```python
from build123d import *

# Parameters (mm, degrees)
F0_W        = 630
F0_H        = 480
F0_R        = 196.5
F1_DEPTH    = 22
F2_T1_DEPTH = 774.568322948
F3_SIZE     = 5


# Not quite as in the source:
# - a fillet or chamfer that OpenCascade refuses, or shapes differently, is made with other operations: its cross-section is extruded or revolved along the edge and cut away or added


with BuildPart() as f1:
    # F0 (on Front) → F1 (new body)
    with BuildSketch(Plane.XZ):
        Rectangle(F0_W, F0_H)
        with Locations((0, -15)):
            Circle(F0_R, mode=Mode.SUBTRACT)
    extrude(amount=F1_DEPTH)

    # F2: fillet of radius 30 on 1 edges, made by hand

    # F2_s2 → F2_t1 (cut)
    with BuildSketch(Plane.YZ.offset(-387.284161474)):
        with BuildLine():
            ThreePointArc((0, 240), (-15.8746727726, 229.252237535), (-22, 211.0863354104))
            Line((-22, 211.0863354104), (-22, 240))
            Line((-22, 240), (0, 240))
        make_face()
    extrude(amount=F2_T1_DEPTH, mode=Mode.SUBTRACT)

    # F3
    f3_edges = [f1.edges().sort_by_distance(p)[0] for p in [
        (-196.5, -22, -15),
    ]]
    chamfer(f3_edges, length=F3_SIZE)


solid = f1.part
```
Geometry check sheet. Reference: the model listing, model coordinates, mm. Coordinates: 2 decimals unless noted, no trailing zeros. Order: outer loops, then holes, each group sorted by start corner. A loop starts at its lowest first (then second) coordinate and runs counter-clockwise, first axis right, second up. Notation, with made-up numbers: M -25.75,56 L -11.75,56 A19 cw -11.75,68 Z; hole C 77.5,71.5 d11. An arc over 180 degrees is marked long. One line per question, with ' | ' between items. Start each with the question number.
Item 1: Cross-section at C-C on y = -11.5. Enter the section's corners in (x, z).
Item 2: Draft check along X on faces 1 (the flat face through (-4, -22, 189)), 2 (the flat face through (-315, -11, -3)), 3 (the conical face through (187.658, -17.243, 44.096)). Enter one of: pulls with the +X half, pulls with the -X half, needs draft (parallel to the pull), parting line crosses it, or undercut.
Item 3: Material ranges on L1, parallel to Z at x = -15.5, y = -7.75; L2, parallel to Z at x = 159, y = -8.5; L3, parallel to X at y = -12.75, z = 61.5, recorded low to high. Write a range as [from, to].
Item 4: Gauge pin test, flat ends, axial feed: pin 1 (12 mm diameter, centred on x = 117, y = -14, fed in from +Z); pin 2 (5 mm diameter, centred on x = 231.5, z = 130, fed in from +Y). Record the tip position at first contact, or that the pin passes through.
Item 5: Cross-section at A-A on z = -15. Enter the section's corners in (x, y), then the cut area to 3 significant figures.
Item 6: Cross-section at B-B on x = 0. Enter the section's corners in (y, z), then the cut area to 3 significant figures.
Findings:
1) outline: M -315,-240 L 315,-240 L 315,233.88 L -315,233.88 Z; hole C 0,-15 d393
2) face 1: needs draft | face 2: pulls with the -X half | face 3: undercut
3) L1: z = [-240, -210.89], [180.89, 236.62] | L2: z = [-240, -130.46], [100.46, 236.14] | L3: x = [-315, -181], [181, 315]
4) pin 1: stops at z = 236.46 | pin 2: stops at y = 0
5) outline: M -315,-22 L -201.5,-22 L -196.5,-17 L -196.5,0 L -315,0 Z; M 196.5,-17 L 201.5,-22 L 315,-22 L 315,0 L 196.5,0 Z | area: 5,190 mm²
6) outline: M -22,-240 L 0,-240 L 0,-211.5 L -17,-211.5 L -22,-216.5 Z; M -22,186.5 L -17,181.5 L 0,181.5 L 0,240 A30 ccw -22,211.09 Z | area: 1,720 mm²
